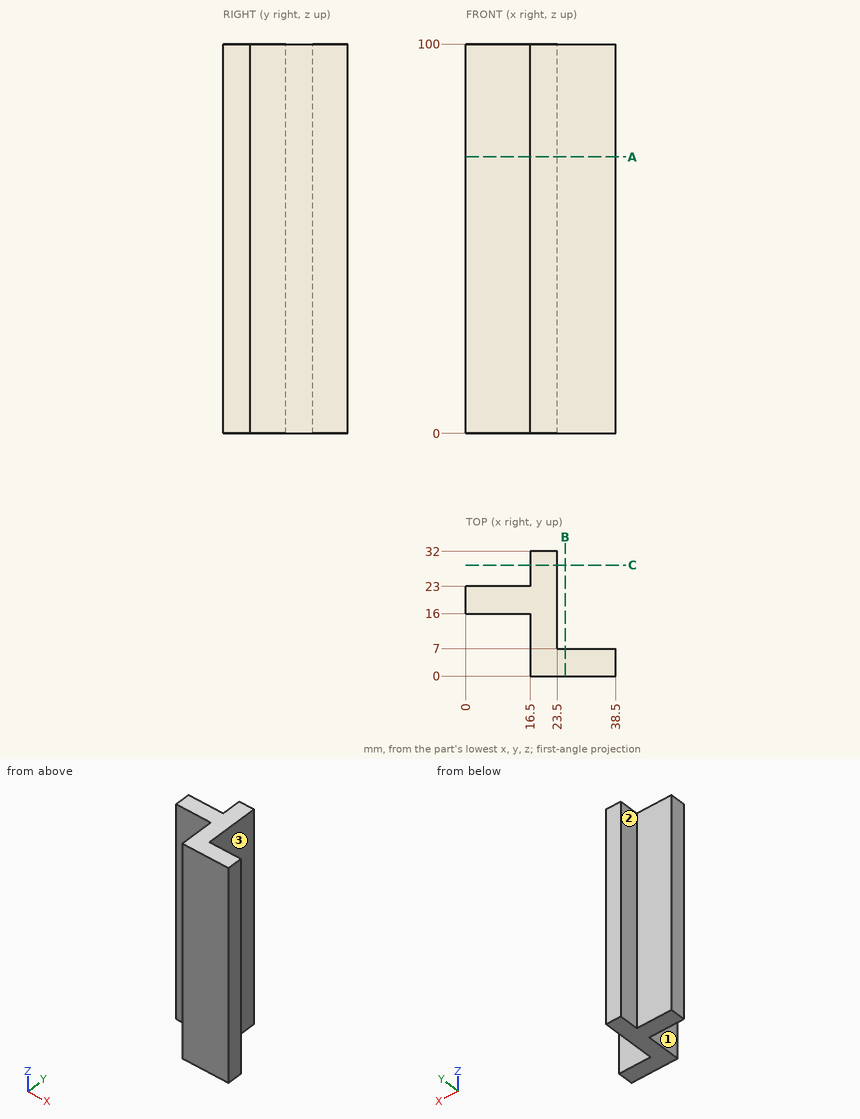
The drawing under review shows one solid part. Ordinate dimensions are in mm from its lowest x, y, z. A direction names the side the tool comes from. Round coordinates to 2 decimals unless told otherwise and drop trailing zeros. Order: outer loops, then holes, each group sorted by start corner. A loop starts at its lowest first (then second) coordinate and runs counter-clockwise, first axis right, second up. Notation, with made-up numbers: (74.25, -5) -> (86.25, -5) arc R20 ccw to (86.25, 17) -> close; hole circle Ø2 at (-19.75, -25.5). An arc over 180 degrees is marked (long way). Use a Markdown table: item, result.
Q1. For line 1 (Y direction, x = 14, z = 80); line 2 (X direction, y = 21.5, z = 24); line 3 (Y direction, x = 36, z = 82.5), list the stretches that pass through material, from the lowest coordinate up.
Values:
| item | result |
|---|---|
| line 1 | y = 16 to 23 |
| line 2 | x = 0 to 23.5 |
| line 3 | y = 0 to 7 |
Q2. Tool access review of the marked faces 1, 2 and 3: name each direction out of +Z, -Z, +X, -X, +Y, -Y from which nothing blocks a thin tool from reaching the whole face with its end or side.
Values:
| item | result |
|---|---|
| face 1 | +Z, -Z, -X, -Y |
| face 2 | +Z, -Z, -X, +Y |
| face 3 | +Z, -Z, +X, +Y |
Q3. We need section C-C on y = 28.5. Write out the cut boundary in (x, z), then the cut area to 3 significant figures.
Values:
| item | result |
|---|---|
| outline | (16.5, 0) -> (23.5, 0) -> (23.5, 100) -> (16.5, 100) -> close |
| area | 700 mm^2 |
Q4. We need section B-B on x = 25.5. Write out the cut boundary in (y, z).
Values:
| item | result |
|---|---|
| outline | (0, 0) -> (7, 0) -> (7, 100) -> (0, 100) -> close |
Q5. We need section A-A on z = 71. Write out the cut boundary in (x, y).
Values:
| item | result |
|---|---|
| outline | (0, 16) -> (16.5, 16) -> (16.5, 0) -> (38.5, 0) -> (38.5, 7) -> (23.5, 7) -> (23.5, 32) -> (16.5, 32) -> (16.5, 23) -> (0, 23) -> close |
Q6. Clearance check with flat-ended pins moving along their axes: P1, Ø12, axis at x = 31.5, z = 35.5, coming from the +Y side; P2, Ø5, axis at y = 6, z = 52, coming from the -X side; P3, Ø8, axis at x = 9, z = 34.5, coming from the -Y side. State where each tip first meets the part, or that it passes through.
Values:
| item | result |
|---|---|
| P1 | stops at y = 7 |
| P2 | stops at x = 16.5 |
| P3 | stops at y = 16 |
